Check sheet for the modelled part. Datum: model origin and axes. Units: mm. Coordinates: 2 decimals unless noted, no trailing zeros. Write each loop counter-clockwise with the first axis right and the second up, starting at its lowest first coordinate (ties: lowest second). Pieces come first, ordered by that corner, then holes. Notation, with made-up numbers: (20.25, 74) - (64.25, 74) arc R36 cw to (64.25, 110) - close; hole circle Ø7 at (85.5, 87.25). An arc over 180 degrees is marked (long way). Answer as CSV lines item,"result". Start each with the question number.
from build123d import *

# Parameters (mm, degrees)
SKETCH1_W                         = 120
SKETCH1_H                         = 53
BOSS_EXTRUDE1_DEPTH               = 3.125
F_1_2_20_TAPPED_HOLE1_D           = 11.50874
F_1_2_20_TAPPED_HOLE1_DEPTH       = 30
F_1_2_20_TAPPED_HOLE1_CSINK_D     = 13.97
F_1_2_20_TAPPED_HOLE1_CSINK_ANGLE = 90
F_1_2_20_TAPPED_HOLE1_TIP         = 3.45757432


with BuildPart() as part:
    # Sketch1 → Boss-Extrude1 (new body)
    with BuildSketch(Plane(origin=(0, 0, 0), x_dir=(1, 0, 0), z_dir=(0, 1, 0))):
        Rectangle(SKETCH1_W, SKETCH1_H)
    extrude(amount=BOSS_EXTRUDE1_DEPTH)

    # 1/2-20 Tapped Hole1
    with Locations(Plane(origin=(0, 3.125, 0), x_dir=(1, 0, 0), z_dir=(0, 1, 0))):
        with Locations((33.5, 0)):
            CounterSinkHole(F_1_2_20_TAPPED_HOLE1_D / 2, F_1_2_20_TAPPED_HOLE1_CSINK_D / 2, depth=F_1_2_20_TAPPED_HOLE1_DEPTH, counter_sink_angle=F_1_2_20_TAPPED_HOLE1_CSINK_ANGLE)
            with Locations((0, 0, -(F_1_2_20_TAPPED_HOLE1_DEPTH + F_1_2_20_TAPPED_HOLE1_TIP / 2))):  # 118° drill point
                Cone(0, F_1_2_20_TAPPED_HOLE1_D / 2, F_1_2_20_TAPPED_HOLE1_TIP, mode=Mode.SUBTRACT)


solid = part.part
(1) Material ranges on probe 1 along Z at (x, y) = (33.5, 1.5); probe 2 along X at (y, z) = (1.2, 3); probe 3 along Z at (x, y) = (31, 1.7), recorded low to high. Write a range as from..to.
(2) Cross-section at A-A on z = 0. Record the boundary of the cut face in (x, y) (3 decimals), plus the area to 3 significant figures.
(3) Cross-section at B-B on x = 33.5. Record the boundary of the cut face in (y, z) (3 decimals), plus the area to 3 significant figures.
(4) Go/stop test with a flat-tipped pin: P1, Ø15, axis at x = 33.5, z = 0, coming from the -Y side. Record where the tip stops, or that it passes through.
(5) Release check for a two-part mould opening along Z. For faces 1 (the face through (-1, 0, 0)), 2 (the face through (-1, 2, -26.5)), 3 (the face through (39.25, 0.93, -0.25)) record: pulls with the +Z half, pulls with the -Z half, needs draft (parallel to the pull), parting line crosses it, or undercut.
(6) Cross-section at C-C on y = 1.25. Record the boundary of the cut face in (x, z).
Checked values:
1,probe 1,"-26.5..-5.75, 5.75..26.5"
1,probe 2,"-60..28.59, 38.41..60"
1,probe 3,"-26.5..-5.18, 5.18..26.5"
2,outline,"(-60, 0) - (27.746, 0) - (27.746, 1.894) - (26.515, 3.125) - (-60, 3.125) - close; (39.254, 0) - (60, 0) - (60, 3.125) - (40.485, 3.125) - (39.254, 1.894) - close"
2,area,"338 mm^2"
3,outline,"(0, -26.5) - (3.125, -26.5) - (3.125, -6.985) - (1.894, -5.754) - (0, -5.754) - close; (0, 5.754) - (1.894, 5.754) - (3.125, 6.985) - (3.125, 26.5) - (0, 26.5) - close"
3,area,"128 mm^2"
4,P1,"y = 0"
5,face 1,"needs draft"
5,face 2,"pulls with the -Z half"
5,face 3,"undercut"
6,outline,"(-60, -26.5) - (60, -26.5) - (60, 26.5) - (-60, 26.5) - close; hole circle Ø11.51 at (33.5, 0)"
